For this review, take the finished solid that the model builds, in its own axes (mm). Face numbers are marked on the shaded views. A direction names the side the tool comes from. Round coordinates to 2 decimals unless told otherwise and drop trailing zeros. Order: outer loops, then holes, each group sorted by start corner. A loop starts at its lowest first (then second) coordinate and runs counter-clockwise, first axis right, second up. Notation, with made-up numbers: M 57.5,73.25 L 103.5,73.25 A20 ccw 103.5,84.25 Z; hole C 61,82 d4. An arc over 180 degrees is marked long. Answer in a Markdown table with one row per item. Add a question column.
```python
from build123d import *

# Parameters (mm, degrees)
SKETCH1_R           = 32
BOSS_EXTRUDE1_DEPTH = 87.72
SKETCH2_W           = 42
SKETCH2_H           = 42
BOSS_EXTRUDE2_DEPTH = 88.78
FILLET2_R           = 0.8
SKETCH3_R           = 10.5
CUT_EXTRUDE1_DEPTH  = 16


with BuildPart() as part:
    # Sketch1 → Boss-Extrude1 (new body)
    with BuildSketch(Plane(origin=(0, 0, 0), x_dir=(0, 0, -1), z_dir=(1, 0, 0))):
        Circle(SKETCH1_R)
    extrude(amount=BOSS_EXTRUDE1_DEPTH)

    # Sketch2 → Boss-Extrude2 (add)
    with BuildSketch(Plane(origin=(87.72, 0, 0), x_dir=(0, 0, -1), z_dir=(1, 0, 0))):
        Rectangle(SKETCH2_W, SKETCH2_H)
    extrude(amount=BOSS_EXTRUDE2_DEPTH)

    # Fillet2
    fillet2_edges = [part.edges().sort_by_distance(p)[0] for p in [
        (87.72, -21, 0),
        (87.72, 0, -21),
        (87.72, 21, 0),
        (87.72, 0, 21),
    ]]
    fillet(fillet2_edges, radius=FILLET2_R)

    # Sketch3 → Cut-Extrude1 (cut)
    with BuildSketch(Plane(origin=(176.5, 0, 0), x_dir=(0, 0, -1), z_dir=(1, 0, 0))):
        Circle(SKETCH3_R)
    extrude(amount=-CUT_EXTRUDE1_DEPTH, mode=Mode.SUBTRACT)


solid = part.part
```
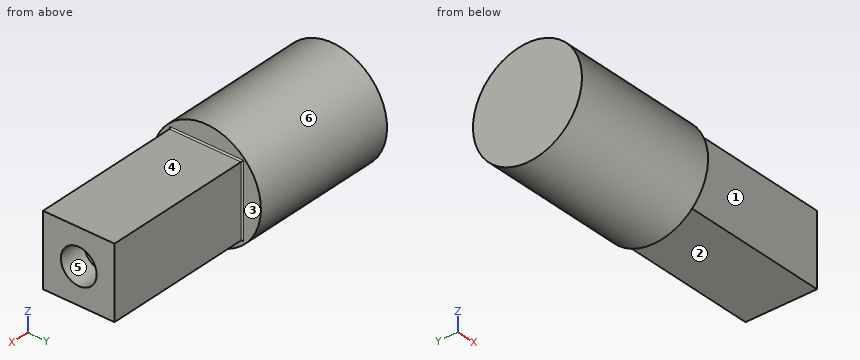
1. For the marked faces 1, 2 and 3, list the 3-axis set-ups (+Z, -Z, +X, -X, +Y, -Y) from which the entire face can be reached by the end or side of a thin tool; tool diameter is ignored.
2. Consider section A-A on y = 0. Write out the cut boundary in (x, z), plus the area to 3 significant figures.
3. Consider section D-D on y = -17.5. Write out the cut boundary in (x, z), plus the area to 3 significant figures.
4. Clearance check with flat-ended pins moving along their axes: pin 1 Ø1 at (x, z) = (69.5, 19) entering from +Y; pin 2 Ø21 at (x, z) = (145.5, -7) entering from -Y; pin 3 Ø6 at (y, z) = (12.5, -21) entering from -X; pin 4 Ø12.5 at (x, y) = (132, 0) entering from +Z. State where each tip first meets the part, or that it passes through.
5. To check wall thickness, follow probe 1 along Y at (x, z) = (172, 0); probe 2 along Y at (x, z) = (146, -10.5); probe 3 along X at (y, z) = (14, -23.5). State the ranges of each line that lie inside material, in increasing order. Write a range as [from, to].
6. Consider section C-C on x = 145.5. Write out the cut boundary in (y, z).
7. The part is to be moulded in two halves that separate along Z. For the marked faces 4, 5 and 6, say which applies: pulls with the +Z half, pulls with the -Z half, needs draft (parallel to the pull), parting line crosses it, or undercut.
Solved:
| question | item | result |
|---|---|---|
| 1 | face 1 | +Z, -Z, +X, -Y |
| 1 | face 2 | -Z, +X, +Y, -Y |
| 1 | face 3 | +X |
| 2 | outline | M 0,-32 L 87.72,-32 L 87.72,-21.8 A0.8 cw 88.52,-21 L 176.5,-21 L 176.5,-10.5 L 160.5,-10.5 L 160.5,10.5 L 176.5,10.5 L 176.5,21 L 88.52,21 A0.8 cw 87.72,21.8 L 87.72,32 L 0,32 Z |
| 2 | area | 9,010 mm^2 |
| 3 | outline | M 0,-26.79 L 87.72,-26.79 L 87.72,-21.8 A0.8 cw 88.52,-21 L 176.5,-21 L 176.5,21 L 88.52,21 A0.8 cw 87.72,21.8 L 87.72,26.79 L 0,26.79 Z |
| 3 | area | 8,430 mm^2 |
| 4 | pin 1 | stops at y = 26.11 |
| 4 | pin 2 | stops at y = -21 |
| 4 | pin 3 | stops at x = 0 |
| 4 | pin 4 | stops at z = 21 |
| 5 | probe 1 | y = [-21, -10.5], [10.5, 21] |
| 5 | probe 2 | y = [-21, 21] |
| 5 | probe 3 | x = [0, 87.72] |
| 6 | outline | M -21,-21 L 21,-21 L 21,21 L -21,21 Z |
| 7 | face 4 | pulls with the +Z half |
| 7 | face 5 | undercut |
| 7 | face 6 | parting line crosses it |
